```python
from build123d import *

# Parameters (mm, degrees)
BOSS_EXTRUDE1_DEPTH       = 6.35
SKETCH2_R                 = 119.0625
SKETCH2_R_2               = 115.2525
CUT_EXTRUDE1_DEPTH        = 2.667
ADVANCEDHOLE1_START       = 4.318
ADVANCEDHOLE1_DEPTH       = 2.032
ADVANCEDHOLE1_2_OUTLINE_R = 1.7272
ADVANCEDHOLE1_2_DEPTH     = 4.318
CIRPATTERN1_COUNT         = 8


# Read off the part's stored shape, not the designer's step: AdvancedHole1
with BuildPart() as part:
    # Sketch1 → Boss-Extrude1 (new body)
    with BuildSketch(Plane(origin=(0, 0, 0), x_dir=(1, 0, 0), z_dir=(0, 1, 0))):
        with BuildLine():
            ThreePointArc((-31.793446259, 122.3), (-48.357791931, 116.746037126), (-63.997797892, 108.960520786))
            Line((-63.997797892, 108.960520786), (-108.960520786, 63.997797892))
            ThreePointArc((-108.960520786, 63.997797892), (-116.746037126, 48.357791931), (-122.3, 31.793446259))
            Line((-122.3, 31.793446259), (-122.3, -31.793446259))
            ThreePointArc((-122.3, -31.793446259), (-116.746037126, -48.357791931), (-108.960520786, -63.997797892))
            Line((-108.960520786, -63.997797892), (-63.997797892, -108.960520786))
            ThreePointArc((-63.997797892, -108.960520786), (-48.357791931, -116.746037126), (-31.793446259, -122.3))
            Line((-31.793446259, -122.3), (31.793446259, -122.3))
            ThreePointArc((31.793446259, -122.3), (48.357791931, -116.746037126), (63.997797892, -108.960520786))
            Line((63.997797892, -108.960520786), (108.960520786, -63.997797892))
            ThreePointArc((108.960520786, -63.997797892), (116.746037126, -48.357791931), (122.3, -31.793446259))
            Line((122.3, -31.793446259), (122.3, 31.793446259))
            ThreePointArc((122.3, 31.793446259), (116.746037126, 48.357791931), (108.960520786, 63.997797892))
            Line((108.960520786, 63.997797892), (63.997797892, 108.960520786))
            ThreePointArc((63.997797892, 108.960520786), (48.357791931, 116.746037126), (31.793446259, 122.3))
            Line((31.793446259, 122.3), (-31.793446259, 122.3))
        make_face()
    extrude(amount=BOSS_EXTRUDE1_DEPTH)

    # Sketch2 → Cut-Extrude1 (cut)
    with BuildSketch(Plane.XZ):
        with Locations(Location((0, 0, 0), (0, 0, 270))):
            Circle(SKETCH2_R)
        with Locations(Location((0, 0, 0), (0, 0, 270))):
            Circle(SKETCH2_R_2, mode=Mode.SUBTRACT)
    extrude(amount=-CUT_EXTRUDE1_DEPTH, mode=Mode.SUBTRACT)

    # AdvancedHole1 outline → AdvancedHole1 (cut)
    with BuildSketch(Plane(origin=(0, 0, 0), x_dir=(1, 0, 0), z_dir=(0, 1, 0)).offset(ADVANCEDHOLE1_START)):
        with BuildLine():
            ThreePointArc((-47.742027192, 116.999196855), (-48.357791931, 116.746037126), (-48.972214314, 116.489636665))
            ThreePointArc((-48.972214314, 116.489636665), (-45.757649346, 110.468737644), (-47.742027192, 116.999196855))
        make_face()
    advancedhole1 = extrude(amount=ADVANCEDHOLE1_DEPTH, mode=Mode.SUBTRACT)

    # AdvancedHole1 2 outline → AdvancedHole1 2 (cut)
    with BuildSketch(Plane(origin=(0, 0, 0), x_dir=(1, 0, 0), z_dir=(0, 1, 0))):
        with Locations((-47.069870839, 113.636720559)):
            Circle(ADVANCEDHOLE1_2_OUTLINE_R)
    advancedhole1_2 = extrude(amount=ADVANCEDHOLE1_2_DEPTH, mode=Mode.SUBTRACT)

    # CirPattern1: AdvancedHole1, AdvancedHole1 2 ×8 about axis
    cirpattern1_axis = Axis((0, 0, 0), (0, 1, 0))
    add([advancedhole1.rotate(cirpattern1_axis, i * 360 / CIRPATTERN1_COUNT) for i in range(1, CIRPATTERN1_COUNT)], mode=Mode.SUBTRACT)
    add([advancedhole1_2.rotate(cirpattern1_axis, i * 360 / CIRPATTERN1_COUNT) for i in range(1, CIRPATTERN1_COUNT)], mode=Mode.SUBTRACT)


solid = part.part
```
CAD build for the part. Positions are in the model's coordinates, mm. A direction names the side the tool comes from. Coordinates: 2 decimals unless noted, no trailing zeros. Loops run counter-clockwise (first coordinate to the right, second up) from the corner with the lowest first, then second, coordinate; pieces in that order, holes last. Notation, with made-up numbers: (18.25, 34) - (44.25, 34) arc R33 ccw to (44.25, 67) - close; hole circle Ø3 at (-40, -34). An arc over 180 degrees is marked (long way). Return JSON: item names as keys, results as strings.
1. Probe L1, parallel to X at y = 1.5, z = 40; L2, parallel to Z at x = 103.5, y = 0.5; L3, parallel to X at y = 1, z = -87.5. List the from-to ranges inside material, lowest first. Write a range as from..to.
Result:
{"L1": "x = -119.87..-112.14, -108.09..108.09, 112.14..119.87", "L2": "z = -69.46..-58.85, -50.7..50.7, 58.85..69.46", "L3": "x = -85.46..-80.74, -75.01..75.01, 80.74..85.46"}
2. 3-axis set-ups, long thin cutter, end or side, ignore diameter. For faces 4 (the flat face through (122.3, 3, 0)), 5 (the flat face through (-47.1, 4.318, 111.5)): which of +Z, -Z, +X, -X, +Y, -Y reach the whole face in a straight line?
Result:
{"face 4": "+Z, -Z, +X, +Y, -Y", "face 5": "+Y"}
3. Band-saw the part on A-A (y = 1). State how many separate pieces and enclosed holes the cut face has, and give its area (3 significant figures).
Result:
{"separate pieces": "2", "enclosed holes": "9", "area": "45,900 mm2"}
4. Band-saw the part on C-C (z = 93.5). Give the cut face in (x, y), and give its area (3 significant figures).
Result:
{"outline": "(-79.46, 0) - (-73.71, 0) - (-73.71, 2.67) - (-67.39, 2.67) - (-67.39, 0) - (67.39, 0) - (67.39, 2.67) - (73.71, 2.67) - (73.71, 0) - (79.46, 0) - (79.46, 6.35) - (-79.46, 6.35) - close", "area": "975 mm2"}
5. Mould opens along Z. For faces 1 (the flat face through (0, 3, -122.3)), 2 (the flat face through (49, 4.318, 114)), 3 (the flat face through (-2, 6.35, -2)) say: released by +Z, released by -Z, zero draft, split by the parting line, or undercut.
Result:
{"face 1": "released by -Z", "face 2": "undercut", "face 3": "zero draft"}
6. Drop flat-ended pins along their axis: pin 1 (3 mm diameter, centred on x = -40, y = 2, fed in from +Z); pin 2 (4 mm diameter, centred on x = 113.64, z = -47.07, fed in from +Y); pin 3 (4 mm diameter, centred on x = 47.07, z = 113.64, fed in from -Y); pin 4 (1 mm diameter, centred on y = 5, z = -34.5, fed in from +X) (3 decimals). Give the stop position or say it passes through.
Result:
{"pin 1": "stops at z = 120.36", "pin 2": "stops at y = 4.32", "pin 3": "stops at y = 0", "pin 4": "stops at x = 121.705"}
7. Band-saw the part on B-B (z = 53.5). Give the cut face in (x, y).
Result:
{"outline": "(-114.48, 0) - (-106.37, 0) - (-106.37, 2.67) - (-102.08, 2.67) - (-102.08, 0) - (102.08, 0) - (102.08, 2.67) - (106.37, 2.67) - (106.37, 0) - (114.48, 0) - (114.48, 6.35) - (-114.48, 6.35) - close"}
